Can you work these out from the model? Positions are in its coordinate system, mm. Face numbers are marked on the shaded views. A direction names the side the tool comes from. Give positions to 0.01 mm unless a question says otherwise; leave off trailing zeros. Order: outer loops, then holes, each group sorted by start corner. A loop starts at its lowest first (then second) coordinate and runs counter-clockwise, first axis right, second up. Notation, with made-up numbers: (56, 3.5) -> (99, 3.5) arc R18 ccw to (99, 22.5) -> close; hole circle Ø6 at (3, 26). An arc over 180 degrees is marked (long way). Answer as CSV lines item,"result".
```python
from build123d import *

# Parameters (mm, degrees)
MIDDLE_COVER_SKETCH_01_W    = 44.37
MIDDLE_COVER_SKETCH_01_H    = 23.06
SALIENTE_EXTRUIR1_DEPTH     = 16.8
VACIADO1_T                  = -1
VACIADO1_THICKNESS_2_FACE_W = 21.06
VACIADO1_THICKNESS_2_FACE_H = 16.8
VACIADO1_THICKNESS_2_DEPTH  = 0.38
VACIADO1_THICKNESS_3_FACE_W = 21.06
VACIADO1_THICKNESS_3_FACE_H = 16.8
VACIADO1_THICKNESS_3_DEPTH  = 0.38
VACIADO1_THICKNESS_4_FACE_W = 43.13
VACIADO1_THICKNESS_4_FACE_H = 16.8
VACIADO1_THICKNESS_4_DEPTH  = 0.08
VACIADO1_THICKNESS_5_FACE_W = 43.13
VACIADO1_THICKNESS_5_FACE_H = 16.8
VACIADO1_THICKNESS_5_DEPTH  = 0.08
REDONDEO1_R                 = 0.5


with BuildPart() as part:
    # Middle-cover-sketch-01 → Saliente-Extruir1 (new body)
    with BuildSketch(Plane(origin=(0, 0, 0), x_dir=(1, 0, 0), z_dir=(0, 1, 0))):
        Rectangle(MIDDLE_COVER_SKETCH_01_W, MIDDLE_COVER_SKETCH_01_H)
    extrude(amount=SALIENTE_EXTRUIR1_DEPTH)

    # Vaciado1
    vaciado1_openings = [part.faces().sort_by_distance(p)[0] for p in [
        (0, 16.8, 0),
        (0, 0, 0),
    ]]
    offset(amount=VACIADO1_T, openings=vaciado1_openings, kind=Kind.INTERSECTION)

    # Vaciado1 thickness 2 face (on inner face of the shell) → Vaciado1 thickness 2 (cut)
    with BuildSketch(Plane(origin=(21.185, 8.4, 0), x_dir=(0, 0, 1), z_dir=(1, 0, 0))):
        Rectangle(VACIADO1_THICKNESS_2_FACE_W, VACIADO1_THICKNESS_2_FACE_H)
    extrude(amount=VACIADO1_THICKNESS_2_DEPTH, mode=Mode.SUBTRACT)

    # Vaciado1 thickness 3 face (on inner face of the shell) → Vaciado1 thickness 3 (cut)
    with BuildSketch(Plane(origin=(-21.185, 8.4, 0), x_dir=(0, 0, -1), z_dir=(-1, 0, 0))):
        Rectangle(VACIADO1_THICKNESS_3_FACE_W, VACIADO1_THICKNESS_3_FACE_H)
    extrude(amount=VACIADO1_THICKNESS_3_DEPTH, mode=Mode.SUBTRACT)

    # Vaciado1 thickness 4 face (on inner face of the shell) → Vaciado1 thickness 4 (cut)
    with BuildSketch(Plane(origin=(0, 8.4, 10.53), x_dir=(1, 0, 0), z_dir=(0, 0, 1))):
        Rectangle(VACIADO1_THICKNESS_4_FACE_W, VACIADO1_THICKNESS_4_FACE_H)
    extrude(amount=VACIADO1_THICKNESS_4_DEPTH, mode=Mode.SUBTRACT)

    # Vaciado1 thickness 5 face (on inner face of the shell) → Vaciado1 thickness 5 (cut)
    with BuildSketch(Plane(origin=(0, 8.4, -10.53), x_dir=(-1, 0, 0), z_dir=(0, 0, -1))):
        Rectangle(VACIADO1_THICKNESS_5_FACE_W, VACIADO1_THICKNESS_5_FACE_H)
    extrude(amount=VACIADO1_THICKNESS_5_DEPTH, mode=Mode.SUBTRACT)

    # Redondeo1
    redondeo1_edges = [part.edges().sort_by_distance(p)[0] for p in [
        (-22.185, 8.4, -11.53),
        (22.185, 8.4, -11.53),
        (22.185, 8.4, 11.53),
        (-22.185, 8.4, 11.53),
    ]]
    fillet(redondeo1_edges, radius=REDONDEO1_R)


solid = part.part
```
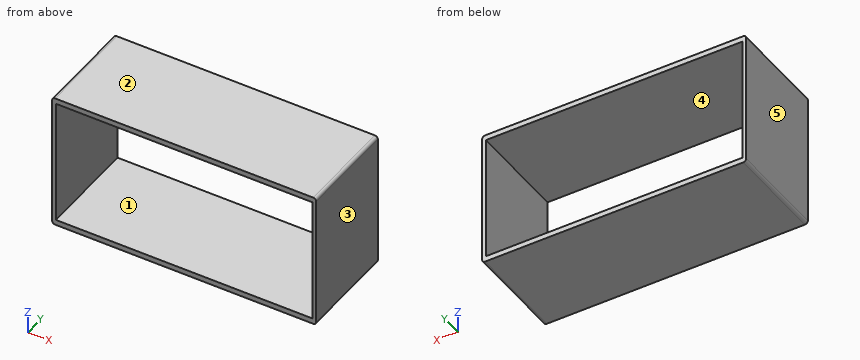
Item 1: We'd pull the mould along Z, two halves only. Please class the marked faces 1, 2 and 3: released by +Z, released by -Z, zero draft, split by the parting line, or undercut.
Numbers:
face 1,"undercut"
face 2,"released by +Z"
face 3,"zero draft"
Item 2: Imagine slicing it at A-A, the plane z = -3. Please give me the cut outline in (x, y) (3 decimals).
Numbers:
outline,"(-22.185, 0) -> (-21.565, 0) -> (-21.565, 16.8) -> (-22.185, 16.8) -> close; (21.565, 0) -> (22.185, 0) -> (22.185, 16.8) -> (21.565, 16.8) -> close"
Item 3: Please list where these lines run through material, in increasing order: line 1 along Z through (x, y) = (2.5, 6.5); line 2 along X through (y, z) = (8.5, 9.5) (3 decimals).
Numbers:
line 1,"z = -11.53 to -10.61, 10.61 to 11.53"
line 2,"x = -22.185 to -21.565, 21.565 to 22.185"
Item 4: Imagine slicing it at C-C, the plane y = 5.25. Please give me the cut outline in (x, z) (3 decimals).
Numbers:
outline,"(-22.185, -11.03) arc R0.5 ccw to (-21.685, -11.53) -> (21.685, -11.53) arc R0.5 ccw to (22.185, -11.03) -> (22.185, 11.03) arc R0.5 ccw to (21.685, 11.53) -> (-21.685, 11.53) arc R0.5 ccw to (-22.185, 11.03) -> close; hole (-21.565, -10.61) -> (21.565, -10.61) -> (21.565, 10.61) -> (-21.565, 10.61) -> close"
Item 5: Imagine slicing it at B-B, the plane x = -4.5. Please give me the cut outline in (y, z).
Numbers:
outline,"(0, -11.53) -> (16.8, -11.53) -> (16.8, -10.61) -> (0, -10.61) -> close; (0, 10.61) -> (16.8, 10.61) -> (16.8, 11.53) -> (0, 11.53) -> close"
Item 6: For the marked faces 4 and 5, which set-ups out of +Z, -Z, +X, -X, +Y, -Y let a thin tool reach every point of the face, with its end or its side?
Numbers:
face 4,"+Y, -Y"
face 5,"+Z, -Z, -X, +Y, -Y"
Item 7: For pin 1 (1.5 mm diameter, centred on x = 6.5, z = 8, fed in from -Y), with a flat end and sliding along its axis, tell me the tip position at first contact or that it passes through.
Numbers:
pin 1,"passes through"
